Could you check a few things on this model? Use its own coordinates, in mm. A direction names the side the tool comes from. Round coordinates to 2 decimals unless told otherwise and drop trailing zeros. Loops run counter-clockwise (first coordinate to the right, second up) from the corner with the lowest first, then second, coordinate; pieces in that order, holes last. Notation, with made-up numbers: (-27, 70.5) - (32, 70.5) arc R24 cw to (32, 84.5) - close; hole circle Ø8 at (-38, 39.25). An arc over 180 degrees is marked (long way). Answer as CSV lines item,"result". Start each with the question number.
1) Which directions (+Z, -Z, +X, -X, +Y, -Y) give clear straight access to the entire face, cutting with the end or side of a thin tool? Please do faces 1 (the face through (-11.923, 3.755, 2.465)), 2 (the face through (13.89, -18.03, 17.98)), 3 (the face through (-20, 27, 23)), 4 (the face through (0, -16, 13)), 5 (the face through (14, -15.43, 2.54)).
2) Suppose I cut it at D-D, the plane y = 15.5. Write out the boundary of the cut face in (x, z), then the cut area to 3 significant figures.
3) Suppose I cut it at C-C, the plane x = 0. Write out the boundary of the cut face in (y, z).
4) I'm going to push flat-ended pins straight in: pin 1 Ø5 at (x, z) = (-18.5, 3) entering from +Y; pin 2 Ø10 at (x, y) = (-8.5, -10.5) entering from -Z; pin 3 Ø9.5 at (x, y) = (0, 0) entering from -Z; pin 4 Ø4 at (y, z) = (28.5, 24) entering from +X. Where does each tip first touch, or does it pass through?
5) Suppose I cut it at A-A, the plane y = 28. Write out the boundary of the cut face in (x, z).
6) Please list where these lines run through material, in increasing order: line 1 along Y through (x, z) = (-15.5, 3.2); line 2 along X through (y, z) = (-15, 6.25); line 3 along Y through (x, z) = (15.5, 24.5).
7) Suppose I cut it at B-B, the plane z = 15. Write out the boundary of the cut face in (x, y), then the cut area to 3 significant figures.
8) We'd pull the mould along Y, two halves only. Please class faces 6 (the face through (20, 28, 23)), 7 (the face through (3, 0, 23)), 8 (the face through (-19, -16, 13)): pulls with the +Y half, pulls with the -Y half, needs draft (parallel to the pull), parting line crosses it, or undercut.
Autodesk Inventor part; units mm, degrees
ref_plane "Plano de trabajo1" through (0, 0, 26) normal (0, 0, -1) x (-1, 0, 0)
ref_plane "YZ Plane" through (0, 0, 0) normal (1, 0, 0) x (0, 1, 0)
ref_plane "XZ Plane" through (0, 0, 0) normal (0, 1, 0) x (-1, 0, 0)
sketch "Boceto1" plane through (0, 0, 0) normal (0, 0, 1) x (1, 0, 0)
  line L0 (-20, 20) -> (20, 20)
  line L1 (20, 20) -> (20, -20)
  line L2 (20, -20) -> (-20, -20)
  line L3 (-20, -20) -> (-20, 20)
  line L4 (6.44, 0) -> (0, 0)
  line L5 (0, 0) -> (0, 3.5859)
  dimension "d0" = 40
  dimension "d1" = 40
extrude "Extrusión1" add sketch "Boceto1" along normal blind 5
sketch "Boceto2" plane through (0, 0, 5) normal (0, 0, 1) x (1, 0, 0)
  circle A0 centre (15.5, 15.5) radius 1.5
  point P0 (0, 0)
  dimension "d4" = 3
  dimension "d5" = 15.5
  dimension "d6" = 15.5
extrude "Extrusión2" cut sketch "Boceto2" against normal through all
pattern_linear "Patrón rectangular1" count 2 spacing 31 along (-1, 0, 0) count 2 spacing 31 along (0, -1, 0) of "Extrusión2"
ref_plane "Plano de trabajo1" through (0, 0, 26) normal (0, 0, -1) x (-1, 0, 0)
sketch "Boceto6" plane through (0, 0, 26) normal (0, 0, -1) x (-1, 0, 0)
  circle A0 centre (15.5, -15.5) radius 1.5
  circle A1 centre (-15.5, -15.5) radius 1.5
  circle A2 centre (15.5, 15.5) radius 1.5
  circle A3 centre (-15.5, 15.5) radius 1.5
  line L0 (20, -20) -> (-20, -20)
  line L1 (-20, -20) -> (-20, 20)
  line L2 (-20, 20) -> (20, 20)
  line L3 (20, 20) -> (20, -20)
  line L4 (20, 20) -> (-20, 20)
  line L5 (-20, 20) -> (-20, 35)
  line L6 (-20, 35) -> (20, 35)
  line L7 (20, 35) -> (20, 20)
  circle A4 centre (-10, 28) radius 2.5
  circle A5 centre (10, 28) radius 2.5
  circle A6 centre (-15.5, -15.5) radius 3
  circle A7 centre (-15.5, 15.5) radius 1.5
  circle A8 centre (-15.5, 15.5) radius 3
  circle A9 centre (15.5, 15.5) radius 1.5
  circle A10 centre (15.5, 15.5) radius 3
  circle A11 centre (15.5, -15.5) radius 1.5
  circle A12 centre (15.5, -15.5) radius 3
  dimension "d31" = 15
  dimension "d32" = 5
  dimension "d33" = 5
  dimension "d34" = 10
  dimension "d35" = 10
  dimension "d36" = 7
  dimension "d37" = 7
  dimension "d40" = 6
  dimension "d41" = 6
  dimension "d42" = 6
  dimension "d43" = 6
extrude "Extrusión5" add sketch "Boceto6" along normal blind 5 contours L0 L1 L2 L3 | L2 L5 L6 L7
sketch "Boceto7" plane through (-20, -20, 0) normal (-1, 0, 0) x (0, 0, 1)
  line L0 (26, 0) -> (26, 55)
  line L1 (5, 40) -> (5, 0)
  line L2 (5, 4) -> (21, 4)
  line L3 (21, 4) -> (21, -1)
  line L4 (21, -1) -> (5, -1)
  line L5 (5, -1) -> (5, 4)
  line L6 (26, 0) -> (21, 0)
  line L7 (0, 0) -> (5, 0)
  line L8 (5, -1) -> (0, -1)
  line L9 (0, -1) -> (0, 0)
  line L10 (0, 0) -> (5, 0)
  line L11 (5, 0) -> (5, -1)
  line L12 (21, -1) -> (26, -1)
  line L13 (26, -1) -> (26, 0)
  line L14 (26, 0) -> (21, 0)
  line L15 (21, 0) -> (21, -1)
  point P0 (0, 20)
  dimension "d48" = 1
  dimension "d49" = 5
extrude "Extrusión6" add sketch "Boceto7" against normal up to surface (40 mm away)
sketch "Boceto8" plane through (0, 0, 26) normal (0, 0, 1) x (1, 0, 0)
  circle A0 centre (-15.5, -15.5) radius 3
  circle A1 centre (15.5, -15.5) radius 3
  point P0 (0, 0)
extrude "Extrusión7" cut sketch "Boceto8" against normal up to surface (21 mm away)
sketch "Boceto9" plane through (-12.542, -16, 5) normal (0, 1, 0) x (1, 0, 0)
  circle A0 centre (2.542, -10) radius 2.5
  circle A1 centre (22.542, -10) radius 2.5
  line L0 (-7.458, -16) -> (-7.458, 0)
  line L1 (32.542, -16) -> (32.542, 0)
  line L2 (-7.458, -21) -> (32.542, -21)
  point P0 (12.542, 5)
  dimension "d52" = 5
  dimension "d53" = 5
  dimension "d54" = 10
  dimension "d55" = 10
  dimension "d56" = 11
  dimension "d57" = 11
extrude "Extrusión8" cut sketch "Boceto9" against normal through all
sketch "Boceto10" plane through (0, 0, 0) normal (0, 0, -1) x (-1, 0, 0)
  circle A0 centre (0, 0) radius 12.5
  dimension "d60" = 25
extrude "Extrusión9" cut sketch "Boceto10" against normal up to surface (5 mm away)
sketch "Boceto11" plane through (-20, 20, 0) normal (0, 1, 0) x (1, 0, 0)
  line L0 (40, 0) -> (0, 0)
  line L1 (0, 0) -> (-3, 0)
  line L2 (-3, 0) -> (-3, -26)
  line L3 (-3, -26) -> (0, -26)
  line L4 (0, -26) -> (0, 0)
  line L5 (40, -26) -> (40, -21)
  line L6 (40, -26) -> (43, -26)
  line L7 (43, -26) -> (43, 0)
  line L8 (43, 0) -> (40, 0)
  line L9 (40, 0) -> (40, -26)
  point P0 (20, 0)
  dimension "d63" = 3
  dimension "d64" = 3
extrude "Extrusión10" add sketch "Boceto11" against normal up to surface (41 mm away)
sketch "Boceto12" plane through (0, 0, 0) normal (0, 0, -1) x (-1, 0, 0)
  circle A0 centre (0, 0) radius 3
  dimension "d67" = 6
extrude "Extrusión11" cut sketch "Boceto12" against normal up to surface (26 mm away)
equation "\"d33\" = d32"
equation "\"d35\" = d34"
equation "\"d36\" = d37"
equation "\"d41\" = d40"
equation "\"d42\" = d40"
equation "\"d43\" = d40"
equation "\"d53\" = d52"
equation "\"d57\" = d56"
equation "\"d64\" = d63"
properties part number "Base Motor Z"
Filled sheet:
1,face 1,"-Z"
1,face 2,"+Z"
1,face 3,"+Z, -Z, -X, +Y"
1,face 4,"+Y"
1,face 5,"+Z, -Z"
2,outline,"(-23, 0) - (-17, 0) - (-17, 5) - (-20, 5) - (-20, 21) - (-18.5, 21) - (-18.5, 26) - (-23, 26) - close; (-14, 0) - (14, 0) - (14, 5) - (-14, 5) - close; (-12.5, 21) - (12.5, 21) - (12.5, 26) - (-12.5, 26) - close; (17, 0) - (23, 0) - (23, 26) - (18.5, 26) - (18.5, 21) - (20, 21) - (20, 5) - (17, 5) - close"
2,area,"466 mm²"
3,outline,"(-21, 0) - (-12.5, 0) - (-12.5, 5) - (-16, 5) - (-16, 21) - (-3, 21) - (-3, 26) - (-21, 26) - close; (3, 21) - (35, 21) - (35, 26) - (3, 26) - close; (12.5, 0) - (20, 0) - (20, 5) - (12.5, 5) - close"
4,pin 1,"y = 20"
4,pin 2,"z = 0"
4,pin 3,"z = 21"
4,pin 4,"x = 20"
5,outline,"(-20, 21) - (-12.5, 21) - (-12.5, 26) - (-20, 26) - close; (-7.5, 21) - (7.5, 21) - (7.5, 26) - (-7.5, 26) - close; (12.5, 21) - (20, 21) - (20, 26) - (12.5, 26) - close"
6,line 1,"-21 to -17, -14 to 14, 17 to 20"
6,line 2,"-23 to -20, 20 to 23"
6,line 3,"-21 to -18.5, -12.5 to 12.5, 18.5 to 35"
7,outline,"(-23, -21) - (-12.5, -21) - (-12.5, -16) - (-12.54, -16) arc R3 cw to (-18.46, -16) - (-20, -16) - (-20, 20) - (-23, 20) - close; (-7.5, -21) - (7.5, -21) - (7.5, -16) - (-7.5, -16) - close; (12.5, -21) - (23, -21) - (23, 20) - (20, 20) - (20, -16) - (18.46, -16) arc R3 cw to (12.54, -16) - (12.5, -16) - close"
7,area,"374 mm²"
8,face 6,"needs draft"
8,face 7,"undercut"
8,face 8,"pulls with the +Y half"
